Read the model definition and answer for the solid it produces. Units are mm, in the model's axes. Coordinates: 2 decimals unless noted, no trailing zeros. Use CSV: the item, a comma, the result in double quotes.
from build123d import *

# Parameters (mm, degrees)
ESTRUSIONE_ESTRUSIONE1_DEPTH = 500


with BuildPart() as part:
    # Schizzo1 → Estrusione-Estrusione1 (new body)
    with BuildSketch(Plane.XY):
        with BuildLine():
            Line((-5, 18.5), (-5, 14))
            Line((-5, 14), (-10.058726211, 14))
            Line((-10.058726211, 14), (-10.058726211, 11.46))
            Line((-10.058726211, 11.46), (-6.085, 7.5))
            Line((-6.085, 7.5), (6.085, 7.5))
            Line((6.085, 7.5), (10.058726211, 11.46))
            Line((10.058726211, 11.46), (10.058726211, 14))
            Line((10.058726211, 14), (5, 14))
            Line((5, 14), (5, 18.5))
            Line((5, 18.5), (5.8, 18.5))
            Line((5.8, 18.5), (5.8, 20))
            Line((5.8, 20), (17.4314, 20))
            ThreePointArc((17.4314, 20), (19.247674478, 19.247674478), (20, 17.4314))
            Line((20, 17.4314), (20, 5.8))
            Line((20, 5.8), (18.5, 5.8))
            Line((18.5, 5.8), (18.5, 5))
            Line((18.5, 5), (14, 5))
            Line((14, 5), (14, 10.058726211))
            Line((14, 10.058726211), (11.46, 10.058726211))
            Line((11.46, 10.058726211), (7.5, 6.085))
            Line((7.5, 6.085), (7.5, -6.085))
            Line((7.5, -6.085), (11.46, -10.058726211))
            Line((11.46, -10.058726211), (14, -10.058726211))
            Line((14, -10.058726211), (14, -5))
            Line((14, -5), (18.5, -5))
            Line((18.5, -5), (18.5, -5.8))
            Line((18.5, -5.8), (20, -5.8))
            Line((20, -5.8), (20, -17.4314))
            ThreePointArc((20, -17.4314), (19.247674478, -19.247674478), (17.4314, -20))
            Line((17.4314, -20), (5.8, -20))
            Line((5.8, -20), (5.8, -18.5))
            Line((5.8, -18.5), (5, -18.5))
            Line((5, -18.5), (5, -14))
            Line((5, -14), (10.058726211, -14))
            Line((10.058726211, -14), (10.058726211, -11.46))
            Line((10.058726211, -11.46), (6.085, -7.5))
            Line((6.085, -7.5), (-6.085, -7.5))
            Line((-6.085, -7.5), (-10.058726211, -11.46))
            Line((-10.058726211, -11.46), (-10.058726211, -14))
            Line((-10.058726211, -14), (-5, -14))
            Line((-5, -14), (-5, -18.5))
            Line((-5, -18.5), (-5.8, -18.5))
            Line((-5.8, -18.5), (-5.8, -20))
            Line((-5.8, -20), (-17.4314, -20))
            ThreePointArc((-17.4314, -20), (-19.247674478, -19.247674478), (-20, -17.4314))
            Line((-20, -17.4314), (-20, -5.8))
            Line((-20, -5.8), (-18.5, -5.8))
            Line((-18.5, -5.8), (-18.5, -5))
            Line((-18.5, -5), (-14, -5))
            Line((-14, -5), (-14, -10.058726211))
            Line((-14, -10.058726211), (-11.46, -10.058726211))
            Line((-11.46, -10.058726211), (-7.5, -6.085))
            Line((-7.5, -6.085), (-7.5, 6.085))
            Line((-7.5, 6.085), (-11.46, 10.058726211))
            Line((-11.46, 10.058726211), (-14, 10.058726211))
            Line((-14, 10.058726211), (-14, 5))
            Line((-14, 5), (-18.5, 5))
            Line((-18.5, 5), (-18.5, 5.8))
            Line((-18.5, 5.8), (-20, 5.8))
            Line((-20, 5.8), (-20, 17.4314))
            ThreePointArc((-20, 17.4314), (-19.247674478, 19.247674478), (-17.4314, 20))
            Line((-17.4314, 20), (-5.8, 20))
            Line((-5.8, 20), (-5.8, 18.5))
            Line((-5.8, 18.5), (-5, 18.5))
        make_face()
        with BuildLine():
            Line((-5.2, 5.2), (-2.26, 5.2))
            Line((-2.26, 5.2), (-1.992985622, 4.585630634))
            ThreePointArc((-1.992985622, 4.585630634), (0, 5), (1.992985622, 4.585630634))
            Line((1.992985622, 4.585630634), (2.26, 5.2))
            Line((2.26, 5.2), (5.2, 5.2))
            Line((5.2, 5.2), (5.2, 2.26))
            Line((5.2, 2.26), (4.585630634, 1.992985622))
            ThreePointArc((4.585630634, 1.992985622), (5, 0), (4.585630634, -1.992985622))
            Line((4.585630634, -1.992985622), (5.2, -2.26))
            Line((5.2, -2.26), (5.2, -5.2))
            Line((5.2, -5.2), (2.26, -5.2))
            Line((2.26, -5.2), (1.992985622, -4.585630634))
            ThreePointArc((1.992985622, -4.585630634), (0, -5), (-1.992985622, -4.585630634))
            Line((-1.992985622, -4.585630634), (-2.26, -5.2))
            Line((-2.26, -5.2), (-5.2, -5.2))
            Line((-5.2, -5.2), (-5.2, -2.26))
            Line((-5.2, -2.26), (-4.585630634, -1.992985622))
            ThreePointArc((-4.585630634, -1.992985622), (-5, 0), (-4.585630634, 1.992985622))
            Line((-4.585630634, 1.992985622), (-5.2, 2.26))
            Line((-5.2, 2.26), (-5.2, 5.2))
        make_face(mode=Mode.SUBTRACT)
        with BuildLine():
            Line((-11.75, 15.5), (-11.75, 14.5))
            ThreePointArc((-11.75, 14.5), (-12.555456352, 12.555456352), (-14.5, 11.75))
            Line((-14.5, 11.75), (-15.5, 11.75))
            Line((-15.5, 11.75), (-15.5, 8))
            Line((-15.5, 8), (-18.5, 8))
            Line((-18.5, 8), (-18.5, 14.5))
            Line((-18.5, 14.5), (-17.25, 14.5))
            ThreePointArc((-17.25, 14.5), (-16.444543648, 16.444543648), (-14.5, 17.25))
            Line((-14.5, 17.25), (-14.5, 18.5))
            Line((-14.5, 18.5), (-8, 18.5))
            Line((-8, 18.5), (-8, 15.5))
            Line((-8, 15.5), (-11.75, 15.5))
        make_face(mode=Mode.SUBTRACT)
        with BuildLine():
            Line((15.5, 11.75), (14.5, 11.75))
            ThreePointArc((14.5, 11.75), (12.555456352, 12.555456352), (11.75, 14.5))
            Line((11.75, 14.5), (11.75, 15.5))
            Line((11.75, 15.5), (8, 15.5))
            Line((8, 15.5), (8, 18.5))
            Line((8, 18.5), (14.5, 18.5))
            Line((14.5, 18.5), (14.5, 17.25))
            ThreePointArc((14.5, 17.25), (16.444543648, 16.444543648), (17.25, 14.5))
            Line((17.25, 14.5), (18.5, 14.5))
            Line((18.5, 14.5), (18.5, 8))
            Line((18.5, 8), (15.5, 8))
            Line((15.5, 8), (15.5, 11.75))
        make_face(mode=Mode.SUBTRACT)
        with BuildLine():
            Line((11.75, -15.5), (11.75, -14.5))
            ThreePointArc((11.75, -14.5), (12.555456352, -12.555456352), (14.5, -11.75))
            Line((14.5, -11.75), (15.5, -11.75))
            Line((15.5, -11.75), (15.5, -8))
            Line((15.5, -8), (18.5, -8))
            Line((18.5, -8), (18.5, -14.5))
            Line((18.5, -14.5), (17.25, -14.5))
            ThreePointArc((17.25, -14.5), (16.444543648, -16.444543648), (14.5, -17.25))
            Line((14.5, -17.25), (14.5, -18.5))
            Line((14.5, -18.5), (8, -18.5))
            Line((8, -18.5), (8, -15.5))
            Line((8, -15.5), (11.75, -15.5))
        make_face(mode=Mode.SUBTRACT)
        with BuildLine():
            Line((-15.5, -11.75), (-14.5, -11.75))
            ThreePointArc((-14.5, -11.75), (-12.555456352, -12.555456352), (-11.75, -14.5))
            Line((-11.75, -14.5), (-11.75, -15.5))
            Line((-11.75, -15.5), (-8, -15.5))
            Line((-8, -15.5), (-8, -18.5))
            Line((-8, -18.5), (-14.5, -18.5))
            Line((-14.5, -18.5), (-14.5, -17.25))
            ThreePointArc((-14.5, -17.25), (-16.444543648, -16.444543648), (-17.25, -14.5))
            Line((-17.25, -14.5), (-18.5, -14.5))
            Line((-18.5, -14.5), (-18.5, -8))
            Line((-18.5, -8), (-15.5, -8))
            Line((-15.5, -8), (-15.5, -11.75))
        make_face(mode=Mode.SUBTRACT)
    extrude(amount=ESTRUSIONE_ESTRUSIONE1_DEPTH)


solid = part.part
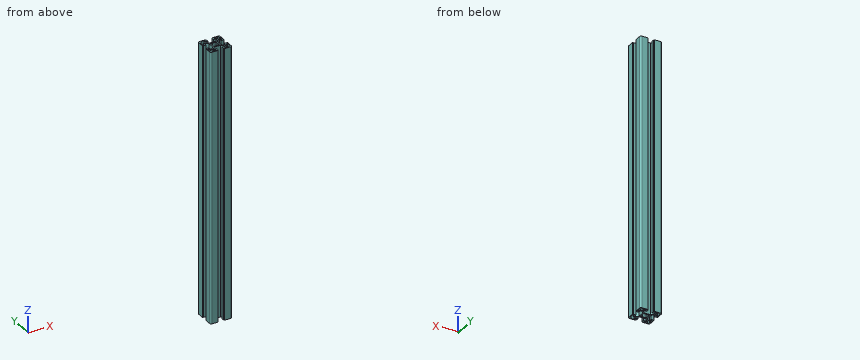
1. A cutting plane is placed at A-A (z = 374.5). Give the number of separate pieces and of enclosed holes in the cut face, and give its area (3 significant figures).
Solutions:
separate pieces,"1"
enclosed holes,"5"
area,"557 mm^2"
2. Find the intervals of material crossed by line 1 along X through (y, z) = (5.5, 460.5); line 2 along X through (y, z) = (17.5, 232); line 3 along Y through (x, z) = (-3.5, 464), in increasing order.
Solutions:
line 1,"x = -18.5 to -14, -7.5 to 7.5, 14 to 18.5"
line 2,"x = -20 to -14.5, -8 to -5, 5 to 8, 14.5 to 20"
line 3,"y = -7.5 to -5.2, 5.2 to 7.5"
3. Each of these flat-tipped pins is pushed along its axis until it touches: pin 1 Ø2.5 at (x, z) = (-3, 171.5) entering from -Y; pin 2 Ø6 at (y, z) = (0, 330.5) entering from -X; pin 3 Ø0.9 at (x, z) = (5, 240.5) entering from -Y. Where does it stop, or does it pass through?
Solutions:
pin 1,"stops at y = -7.5"
pin 2,"stops at x = -7.5"
pin 3,"stops at y = -18.5"
